The listing builds one solid part. Answer for the finished solid, in the listing's coordinates (mm). A direction names the side the tool comes from. Round coordinates to 2 decimals unless told otherwise and drop trailing zeros. Write each loop counter-clockwise with the first axis right and the second up, starting at its lowest first coordinate (ties: lowest second). Pieces come first, ordered by that corner, then holes.
Item 1: Find section C-C on z = -1. Give the vertices of the cut face in (x, y), then the cut area to 3 significant figures.
Item 2: Find the intervals of material crossed by probe 1 along Y at (x, z) = (0, 2); probe 2 along Z at (x, y) = (-4.75, 1.5) (1 decimal); probe 3 along Y at (x, z) = (0, 0.75), in increasing order.
Item 3: Each of these flat-tipped pins is pushed along its axis until it touches: pin 1 (3 mm diameter, centred on y = -2, z = 0, fed in from -X); pin 2 (2 mm diameter, centred on x = -5, z = 0, fed in from +Y); pin 3 (1 mm diameter, centred on y = -1, z = 2, fed in from +X). Where does it stop, or does it pass through?
Item 4: A tool of negligible diameter and unlimited length cuts with its end or side. For faces 1 (the face through (3, -3, 3.175)), 2 (the face through (-2, -5, 1.588)), from which of +Z, -Z, +X, -X, +Y, -Y can it reach the whole face along a straight path? Write none if from no direction.
Item 5: For a pull along Y with two mould halves and no side action, classify faces 3 (the face through (2, -3, -3.175)), 4 (the face through (1.47, -2.83, 0.04)), 5 (the face through (-1.38, -6.2, 2.39)) as +Y half, -Y half, draft (parallel to the pull), parting line (faces both ways), or undercut.
Item 6: Find section D-D on z = 2.75. Give the vertices of the cut face in (x, y), then the cut area to 3 significant figures.
```python
from build123d import *

# Parameters (mm, degrees)
BOSS_EXTRUDE1_START = 3.175
SKETCH3_R           = 6.35
SKETCH3_R_2         = 3.1877
BOSS_EXTRUDE1_DEPTH = 1.5875
BOSS_EXTRUDE2_START = 1.5875
SKETCH4_R           = 4.7879
SKETCH4_R_2         = 3.1877
BOSS_EXTRUDE2_DEPTH = 4.7625
CHAMFER1_SIZE       = 0.095631


with BuildPart() as part:
    # Sketch3 → Boss-Extrude1 (new body)
    with BuildSketch(Plane.XY.offset(BOSS_EXTRUDE1_START)):
        Circle(SKETCH3_R)
        Circle(SKETCH3_R_2, mode=Mode.SUBTRACT)
    extrude(amount=-BOSS_EXTRUDE1_DEPTH)

    # Sketch4 → Boss-Extrude2 (add)
    with BuildSketch(Plane.XY.offset(BOSS_EXTRUDE2_START)):
        Circle(SKETCH4_R)
        Circle(SKETCH4_R_2, mode=Mode.SUBTRACT)
    extrude(amount=-BOSS_EXTRUDE2_DEPTH)

    # Chamfer1
    chamfer1_edges = [part.edges().sort_by_distance(p)[0] for p in [
        (-3.1877, 0, -3.175),
        (-4.7879, 0, 1.5875),
        (-6.35, 0, 3.175),
        (-6.35, 0, 1.5875),
        (-3.1877, 0, 3.175),
        (-4.7879, 0, -3.175),
    ]]
    chamfer(chamfer1_edges, length=CHAMFER1_SIZE)


solid = part.part
```
Check values:
1. outline: circle Ø9.58 at (0, 0); hole circle Ø6.38 at (0, 0)
1. area: 40.1 mm2
2. probe 1: y = -6.35 to -3.19, 3.19 to 6.35
2. probe 2: z = 1.6 to 3.2
2. probe 3: y = -4.79 to -3.19, 3.19 to 4.79
3. pin 1: stops at x = -4.76
3. pin 2: stops at y = 2.63
3. pin 3: stops at x = 6.33
4. face 1: +Z, +X, -X, +Y, -Y
4. face 2: -Z
5. face 3: draft
5. face 4: undercut
5. face 5: parting line
6. outline: circle Ø12.7 at (0, 0); hole circle Ø6.38 at (0, 0)
6. area: 94.8 mm2
